The listing builds one solid part. Answer for the finished solid, in the listing's coordinates (mm). Coordinates: 2 decimals unless noted, no trailing zeros. Order: outer loops, then holes, each group sorted by start corner. A loop starts at its lowest first (then second) coordinate and runs counter-clockwise, first axis right, second up.
from build123d import *

# Parameters (mm, degrees)
SKETCH1_R           = 52.07
SKETCH1_R_2         = 1.575
BOSS_EXTRUDE1_DEPTH = 3.175
SKETCH2_R           = 3.2639
CUT_EXTRUDE1_DEPTH  = 4.175
SKETCH3_R           = 3.2639
CUT_EXTRUDE2_DEPTH  = 4.175
CUT_EXTRUDE3_DEPTH  = 4.175
CUT_EXTRUDE4_DEPTH  = 4.175


with BuildPart() as part:
    # Sketch1 → Boss-Extrude1 (new body)
    with BuildSketch(Plane(origin=(0, 0, 0), x_dir=(1, 0, 0), z_dir=(0, 1, 0))):
        with BuildLine():
            Line((387.35, 76.2), (387.35, -76.2))
            Line((387.35, -76.2), (454.496015193, -111.125))
            Line((454.496015193, -111.125), (454.496015193, -174.625))
            ThreePointArc((454.496015193, -174.625), (435.897295799, -219.526280605), (390.996015193, -238.125))
            Line((390.996015193, -238.125), (213.196015193, -238.125))
            Line((213.196015193, -238.125), (103.210788913, -174.625))
            Line((103.210788913, -174.625), (-103.210788913, -174.625))
            Line((-103.210788913, -174.625), (-213.196015193, -238.125))
            Line((-213.196015193, -238.125), (-390.996015193, -238.125))
            ThreePointArc((-390.996015193, -238.125), (-435.897295799, -219.526280605), (-454.496015193, -174.625))
            Line((-454.496015193, -174.625), (-454.496015193, -111.125))
            Line((-454.496015193, -111.125), (-387.35, -76.2))
            Line((-387.35, -76.2), (-387.35, 76.2))
            Line((-387.35, 76.2), (-454.496015193, 111.125))
            Line((-454.496015193, 111.125), (-454.496015193, 174.625))
            ThreePointArc((-454.496015193, 174.625), (-435.897295799, 219.526280605), (-390.996015193, 238.125))
            Line((-390.996015193, 238.125), (-213.196015193, 238.125))
            Line((-213.196015193, 238.125), (-103.210788913, 174.625))
            Line((-103.210788913, 174.625), (103.210788913, 174.625))
            Line((103.210788913, 174.625), (213.196015193, 238.125))
            Line((213.196015193, 238.125), (390.996015193, 238.125))
            ThreePointArc((390.996015193, 238.125), (435.897295799, 219.526280605), (454.496015193, 174.625))
            Line((454.496015193, 174.625), (454.496015193, 111.125))
            Line((454.496015193, 111.125), (387.35, 76.2))
        make_face()
        with Locations((273.05, 149.225)):
            Circle(SKETCH1_R, mode=Mode.SUBTRACT)
        with Locations((273.05, -149.225)):
            Circle(SKETCH1_R, mode=Mode.SUBTRACT)
        with Locations((-273.05, 149.225)):
            Circle(SKETCH1_R, mode=Mode.SUBTRACT)
        with Locations((-273.05, -149.225)):
            Circle(SKETCH1_R, mode=Mode.SUBTRACT)
        with Locations((382.768773857, 179.375)):
            Circle(SKETCH1_R_2, mode=Mode.SUBTRACT)
        with Locations((395.746015193, 182.852241336)):
            Circle(SKETCH1_R_2, mode=Mode.SUBTRACT)
        with Locations((399.223256529, 169.875)):
            Circle(SKETCH1_R_2, mode=Mode.SUBTRACT)
        with Locations((386.246015193, 166.397758664)):
            Circle(SKETCH1_R_2, mode=Mode.SUBTRACT)
        with Locations((386.246015193, -166.397758664)):
            Circle(SKETCH1_R_2, mode=Mode.SUBTRACT)
        with Locations((399.223256529, -169.875)):
            Circle(SKETCH1_R_2, mode=Mode.SUBTRACT)
        with Locations((395.746015193, -182.852241336)):
            Circle(SKETCH1_R_2, mode=Mode.SUBTRACT)
        with Locations((382.768773857, -179.375)):
            Circle(SKETCH1_R_2, mode=Mode.SUBTRACT)
        with Locations((-399.223256529, 169.875)):
            Circle(SKETCH1_R_2, mode=Mode.SUBTRACT)
        with Locations((-395.746015193, 182.852241336)):
            Circle(SKETCH1_R_2, mode=Mode.SUBTRACT)
        with Locations((-382.768773857, 179.375)):
            Circle(SKETCH1_R_2, mode=Mode.SUBTRACT)
        with Locations((-386.246015193, 166.397758664)):
            Circle(SKETCH1_R_2, mode=Mode.SUBTRACT)
        with Locations((-386.246015193, -166.397758664)):
            Circle(SKETCH1_R_2, mode=Mode.SUBTRACT)
        with Locations((-399.223256529, -169.875)):
            Circle(SKETCH1_R_2, mode=Mode.SUBTRACT)
        with Locations((-382.768773857, -179.375)):
            Circle(SKETCH1_R_2, mode=Mode.SUBTRACT)
        with Locations((-395.746015193, -182.852241336)):
            Circle(SKETCH1_R_2, mode=Mode.SUBTRACT)
    extrude(amount=BOSS_EXTRUDE1_DEPTH)

    # Sketch2 → Cut-Extrude1 (cut, through all)
    with BuildSketch(Plane(origin=(0, 3.175, 0), x_dir=(1, 0, 0), z_dir=(0, 1, 0))):
        with Locations((346.075, 95.25)):
            Circle(SKETCH2_R)
        with Locations((346.075, 57.15)):
            Circle(SKETCH2_R)
        with Locations((212.725, 95.25)):
            Circle(SKETCH2_R)
        with Locations((174.625, 95.25)):
            Circle(SKETCH2_R)
        with Locations((15.875, 95.25)):
            Circle(SKETCH2_R)
        with Locations((-22.225, 95.25)):
            Circle(SKETCH2_R)
        with Locations((-22.225, 57.15)):
            Circle(SKETCH2_R)
        with Locations((346.075, -57.15)):
            Circle(SKETCH2_R)
        with Locations((346.075, -95.25)):
            Circle(SKETCH2_R)
        with Locations((212.725, -95.25)):
            Circle(SKETCH2_R)
        with Locations((174.625, -95.25)):
            Circle(SKETCH2_R)
        with Locations((15.875, -95.25)):
            Circle(SKETCH2_R)
        with Locations((-22.225, -95.25)):
            Circle(SKETCH2_R)
        with Locations((-22.225, -57.15)):
            Circle(SKETCH2_R)
        with BuildLine():
            Line((0, 85.725), (323.85, 85.725))
            ThreePointArc((323.85, 85.725), (332.830256121, 82.005256121), (336.55, 73.025))
            Line((336.55, 73.025), (336.55, -73.025))
            ThreePointArc((336.55, -73.025), (332.830256121, -82.005256121), (323.85, -85.725))
            Line((323.85, -85.725), (0, -85.725))
            ThreePointArc((0, -85.725), (-8.980256121, -82.005256121), (-12.7, -73.025))
            Line((-12.7, -73.025), (-12.7, 73.025))
            ThreePointArc((-12.7, 73.025), (-8.980256121, 82.005256121), (0, 85.725))
        make_face()
    extrude(amount=-CUT_EXTRUDE1_DEPTH, mode=Mode.SUBTRACT)

    # Sketch3 → Cut-Extrude2 (cut, through all)
    with BuildSketch(Plane(origin=(0, 3.175, 0), x_dir=(1, 0, 0), z_dir=(0, 1, 0))):
        with Locations((184.362499956, 149.225)):
            Circle(SKETCH3_R)
        with Locations((-250.095985926, 63.559453238)):
            Circle(SKETCH3_R)
        with Locations((184.362499956, -149.225)):
            Circle(SKETCH3_R)
        with Locations((-250.095985926, -63.559453238)):
            Circle(SKETCH3_R)
        with Locations((216.336503702, 173.759515988)):
            Circle(SKETCH3_R)
        with Locations((216.336503702, 124.690484012)):
            Circle(SKETCH3_R)
        with Locations((-282.069989672, 88.093969226)):
            Circle(SKETCH3_R)
        with Locations((-234.672944416, 100.793969226)):
            Circle(SKETCH3_R)
        with Locations((216.336503702, -124.690484012)):
            Circle(SKETCH3_R)
        with Locations((216.336503702, -173.759515988)):
            Circle(SKETCH3_R)
        with Locations((-234.672944416, -100.793969226)):
            Circle(SKETCH3_R)
        with Locations((-282.069989672, -88.093969226)):
            Circle(SKETCH3_R)
    extrude(amount=-CUT_EXTRUDE2_DEPTH, mode=Mode.SUBTRACT)

    # Sketch4 → Cut-Extrude3 (cut, through all)
    with BuildSketch(Plane(origin=(0, 3.175, 0), x_dir=(1, 0, 0), z_dir=(0, 1, 0))):
        with BuildLine():
            Line((-344.17, 25.4), (-344.17, -25.4))
            ThreePointArc((-344.17, -25.4), (-356.87, -38.1), (-369.57, -25.4))
            Line((-369.57, -25.4), (-369.57, 25.4))
            ThreePointArc((-369.57, 25.4), (-356.87, 38.1), (-344.17, 25.4))
        make_face()
        with BuildLine():
            Line((344.17, 25.4), (344.17, -25.4))
            ThreePointArc((344.17, -25.4), (356.87, -38.1), (369.57, -25.4))
            Line((369.57, -25.4), (369.57, 25.4))
            ThreePointArc((369.57, 25.4), (356.87, 38.1), (344.17, 25.4))
        make_face()
    extrude(amount=-CUT_EXTRUDE3_DEPTH, mode=Mode.SUBTRACT)

    # Sketch5 → Cut-Extrude4 (cut, through all)
    with BuildSketch(Plane(origin=(0, 3.175, 0), x_dir=(1, 0, 0), z_dir=(0, 1, 0))):
        with BuildLine():
            Line((-25.4, 149.225), (25.4, 149.225))
            ThreePointArc((25.4, 149.225), (38.1, 136.525), (25.4, 123.825))
            Line((25.4, 123.825), (-25.4, 123.825))
            ThreePointArc((-25.4, 123.825), (-38.1, 136.525), (-25.4, 149.225))
        make_face()
        with BuildLine():
            Line((-25.4, -149.225), (25.4, -149.225))
            ThreePointArc((25.4, -149.225), (38.1, -136.525), (25.4, -123.825))
            Line((25.4, -123.825), (-25.4, -123.825))
            ThreePointArc((-25.4, -123.825), (-38.1, -136.525), (-25.4, -149.225))
        make_face()
    extrude(amount=-CUT_EXTRUDE4_DEPTH, mode=Mode.SUBTRACT)


solid = part.part
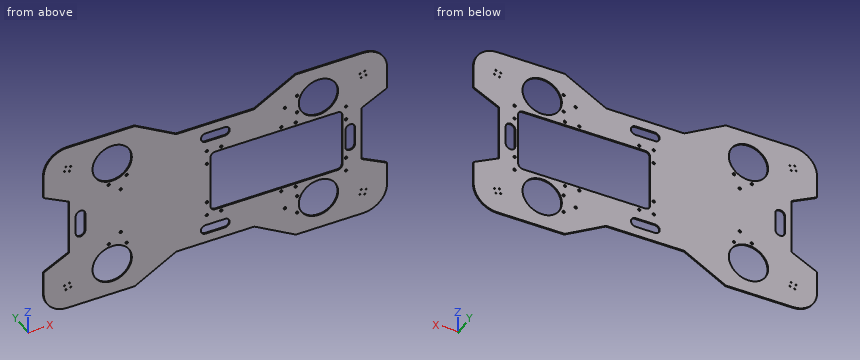
1) Section A-A (x = 73.5) is taken. Give the vertices of the cut face in (y, z) (3 decimals).
2) Each of these flat-tipped pins is pushed along its axis until it touches: P1, Ø1.5, axis at y = 2.5, z = 179, coming from the -X side; P2, Ø8.5, axis at x = -234.67, z = 100.79, coming from the -Y side; P3, Ø1, axis at y = 1, z = -36, coming from the +X side; P4, Ø1.5, axis at y = 2.5, z = -109.5, coming from the +X side. Where does it stop, or does it pass through?
3) Section D-D (y = 0.6) is taken. Give the number of separate pieces and of enclosed holes in the cut face, then the cut area to 3 significant figures.
4) Section C-C (x = -356.87) is taken. Give the vertices of the cut face in (y, z) (3 decimals), then the cut area to 3 significant figures.
5) Section B-B (x = -262) is taken. Give the vertices of the cut face in (y, z) (3 decimals).
6) Consider L1, parallel to X at y = 2.9, z = -57; L2, parallel to X at y = 1.95, z = -10; L3, parallel to Z at x = 226, y = 1.6 (3 decimals). Determine where each line is inside the solid, lowest interval first.
Filled sheet:
1. outline: (0, -174.625) - (3.175, -174.625) - (3.175, -85.725) - (0, -85.725) - close; (0, 85.725) - (3.175, 85.725) - (3.175, 174.625) - (0, 174.625) - close
2. P1: stops at x = -454.39
2. P2: stops at y = 0
2. P3: stops at x = 387.35
2. P4: stops at x = 452.81
3. separate pieces: 1
3. enclosed holes: 51
3. area: 262,000 mm2
4. outline: (0, -238.125) - (3.175, -238.125) - (3.175, -38.1) - (0, -38.1) - close; (0, 38.1) - (3.175, 38.1) - (3.175, 238.125) - (0, 238.125) - close
4. area: 1,270 mm2
5. outline: (0, -238.125) - (3.175, -238.125) - (3.175, -200.109) - (0, -200.109) - close; (0, -98.341) - (3.175, -98.341) - (3.175, 98.341) - (0, 98.341) - close; (0, 200.109) - (3.175, 200.109) - (3.175, 238.125) - (0, 238.125) - close
6. L1: x = -387.35 to -25.49, -18.96 to -12.7, 336.55 to 342.81, 349.34 to 387.35
6. L2: x = -387.35 to -369.57, -344.17 to -12.7, 336.55 to 344.17, 369.57 to 387.35
6. L3: z = -238.125 to -171.532, -126.918 to -85.725, 85.725 to 126.918, 171.532 to 238.125
